from build123d import *

# Parameters (mm, degrees)
F1_DEPTH = 95.8433821797
F0_W     = 16.1665417254
F0_H     = 108.9052408934
F2_DEPTH = 48.777140677
F3_T     = -2.54


with BuildPart() as f1:
    # F0 (on Top) → F1 (new body)
    with BuildSketch(Plane.XY):
        Polygon((37.7709232271, 57.3377944529), (-31.9253392518, 57.3377944529), (-31.9253392518, -50.960008055), (-31.9253392518, -51.6111589968), (37.7709232271, -51.6111589968), (37.7709232271, -51.5674464405), align=None)
    extrude(amount=F1_DEPTH)

    # F0 (on Top) → F2 (join)
    with BuildSketch(Plane.XY):
        Polygon((-31.9253392518, -50.960008055), (-31.9253392518, 57.3377944529), (-48.7250611186, 57.3377944529), (-48.7250611186, -12.884741649), (-48.7250611186, -50.960008055), align=None)
        with Locations((45.8541940898, 2.8851740062)):
            Rectangle(F0_W, F0_H)
    extrude(amount=F2_DEPTH)

    # F3
    f3_openings = [f1.faces().sort_by_distance(p)[0] for p in [
        (-48.725061, 3.188893, 24.38857),
    ]]
    offset(amount=F3_T, openings=f3_openings, kind=Kind.INTERSECTION)


solid = f1.part
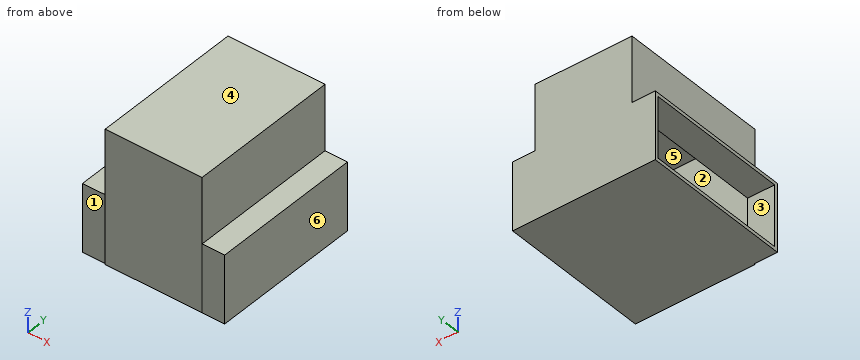
The model under review builds one solid part; all positions refer to its coordinate system, in mm. Face numbers are marked on the shaded views. A direction names the side the tool comes from. Give positions to 0.01 mm unless a question says otherwise; leave off trailing zeros. Order: outer loops, then holes, each group sorted by start corner. A loop starts at its lowest first (then second) coordinate and runs counter-clockwise, first axis right, second up. Notation, with made-up numbers: M -10.5,11.5 L 10.5,11.5 A19 ccw 10.5,17.5 Z; hole C 29.5,5 d3. An arc over 180 degrees is marked long. Answer in a Markdown table with one row per item. Add a question column.
1. Add section D-D on z = 20.5. State the section outline as (x, y) points.
2. Add section B-B on z = 80.5. State the section outline as (x, y) points, plus the area to 3 significant figures.
3. For pin 1 Ø18 at (x, y) = (49, 22) entering from +Z; pin 2 Ø6 at (x, y) = (-37.5, -16.5) entering from -Z; pin 3 Ø8 at (x, z) = (46, 15) entering from -Y; pin 4 Ø12 at (y, z) = (-29, 31.5) entering from -X, all flat-tipped, find the tip position at first contact; note any pin that passes through.
4. Add section A-A on x = 29.5. State the section outline as (y, z) points, plus the area to 3 significant figures.
5. Machinability: for the marked faces 1, 2 and 3, which of the approach directions +Z, -Z, +X, -X, +Y, -Y give a long, thin tool a straight path to every point of the face, cutting with its end or side? Answer none if there is none.
6. Mouldability with a two-part tool opening along X and no side actions: class the marked faces 4, 5 and 6 as released by +X, released by -X, zero draft, split by the parting line, or undercut.
7. To check wall thickness, follow line 1 along Z through (x, y) = (9.5, -23.5); line 2 along Y through (x, z) = (19, 21.5); line 3 along X through (y, z) = (20, 60.5). State the ranges of each line that lie inside material, in increasing order.
8. Add section C-C on y = 38.5. State the section outline as (x, z) points.
The answers:
| question | item | result |
|---|---|---|
| 1 | outline | M -48.73,-50.96 L -31.93,-50.96 L -31.93,-51.61 L 37.77,-51.61 L 37.77,-51.57 L 53.94,-51.57 L 53.94,57.34 L -48.73,57.34 L -48.73,54.8 L 51.4,54.8 L 51.4,-49.03 L 35.23,-49.03 L 35.23,-49.07 L -29.39,-49.07 L -29.39,-48.42 L -48.73,-48.42 Z |
| 2 | outline | M -31.93,-51.61 L 37.77,-51.61 L 37.77,57.34 L -31.93,57.34 Z; hole M -29.39,-49.07 L 35.23,-49.07 L 35.23,54.8 L -29.39,54.8 Z |
| 2 | area | 882 mm2 |
| 3 | pin 1 | z = 48.78 |
| 3 | pin 2 | z = 0 |
| 3 | pin 3 | y = -51.57 |
| 3 | pin 4 | x = 51.4 |
| 4 | outline | M -51.61,0 L 57.34,0 L 57.34,95.84 L -51.61,95.84 Z; hole M -49.07,2.54 L 54.8,2.54 L 54.8,93.3 L -49.07,93.3 Z |
| 4 | area | 1,010 mm2 |
| 5 | face 1 | +Z, -Z, -X, -Y |
| 5 | face 2 | none |
| 5 | face 3 | -X |
| 6 | face 4 | zero draft |
| 6 | face 5 | undercut |
| 6 | face 6 | released by +X |
| 7 | line 1 | 0 to 2.54, 93.3 to 95.84 |
| 7 | line 2 | -51.61 to -49.07, 54.8 to 57.34 |
| 7 | line 3 | -31.93 to -29.39, 35.23 to 37.77 |
| 8 | outline | M -48.73,0 L 53.94,0 L 53.94,48.78 L 37.77,48.78 L 37.77,95.84 L -31.93,95.84 L -31.93,48.78 L -48.73,48.78 L -48.73,46.24 L -29.39,46.24 L -29.39,93.3 L 35.23,93.3 L 35.23,46.24 L 51.4,46.24 L 51.4,2.54 L -48.73,2.54 Z |
